```python
from build123d import *

# Parameters (mm, degrees)
REVOLVE1_ANGLE      = 180
SKETCH4_R           = 50
BOSS_EXTRUDE1_DEPTH = 7
SKETCH5_R           = 4
SKETCH5_R_2         = 1.5
BOSS_EXTRUDE2_DEPTH = 10
SKETCH6_R           = 27.5
CUT_EXTRUDE1_DEPTH  = 10
BOSS_EXTRUDE3_DEPTH = 7
SKETCH8_R           = 3
BOSS_EXTRUDE4_DEPTH = 15
BOSS_EXTRUDE5_DEPTH = 10


with BuildPart() as part:
    # Sketch1 → Revolve1 (revolve)
    with BuildSketch(Plane(origin=(0, 0, 0), x_dir=(1, 0, 0), z_dir=(0, 1, 0))):
        with BuildLine():
            Line((1.491717845, 54.979766986), (-1.491717845, -54.979766986))
            ThreePointArc((-1.491717845, -54.979766986), (54.979766986, -1.491717845), (1.491717845, 54.979766986))
        make_face()
    revolve(axis=Axis((1.491717845, 0, -54.979766986), (-0.027122143, 0, 0.999632127)), revolution_arc=REVOLVE1_ANGLE)

    # Sketch2 → Cut-Revolve1 (revolve, cut)
    with BuildSketch(Plane.XZ):
        with BuildLine():
            Line((49.980692072, 1.389395568), (-49.980692072, -1.389395568))
            ThreePointArc((-49.980692072, -1.389395568), (-1.389395568, 49.980692072), (49.980692072, 1.389395568))
        make_face()
    revolve(axis=Axis((49.980692072, 0, 1.389395568), (-0.999613841, 0, -0.027787911)), mode=Mode.SUBTRACT)

    # Sketch4 → Boss-Extrude1 (add)
    with BuildSketch(Plane.XZ):
        Circle(SKETCH4_R)
    extrude(amount=-BOSS_EXTRUDE1_DEPTH)

    # Sketch5 → Boss-Extrude2 (add)
    with BuildSketch(Plane.XZ):
        with Locations((0, 35)):
            Circle(SKETCH5_R)
        with Locations((0, 35)):
            Circle(SKETCH5_R_2, mode=Mode.SUBTRACT)
        with Locations((30.310889132, -17.5)):
            Circle(SKETCH5_R)
        with Locations((30.310889132, -17.5)):
            Circle(SKETCH5_R_2, mode=Mode.SUBTRACT)
        with Locations((-30.310889132, -17.5)):
            Circle(SKETCH5_R)
        with Locations((-30.310889132, -17.5)):
            Circle(SKETCH5_R_2, mode=Mode.SUBTRACT)
    extrude(amount=BOSS_EXTRUDE2_DEPTH)

    # Sketch6 → Cut-Extrude1 (cut)
    with BuildSketch(Plane.XZ):
        Circle(SKETCH6_R)
    extrude(amount=-CUT_EXTRUDE1_DEPTH, mode=Mode.SUBTRACT)

    # Sketch7 → Boss-Extrude3 (add)
    with BuildSketch(Plane.XZ):
        with BuildLine():
            Line((-29.59626463, 3), (-6.873863542, 3))
            ThreePointArc((-6.873863542, 3), (-5.303300859, 5.303300859), (-3, 6.873863542))
            Line((-3, 6.873863542), (-3, 29.076054117))
            Line((-3, 29.076054117), (3, 29.076054117))
            Line((3, 29.076054117), (3, 6.873863542))
            ThreePointArc((3, 6.873863542), (5.303300859, 5.303300859), (6.873863542, 3))
            Line((6.873863542, 3), (29.260564873, 3))
            Line((29.260564873, 3), (29.260564873, -3))
            Line((29.260564873, -3), (6.873863542, -3))
            ThreePointArc((6.873863542, -3), (5.303300859, -5.303300859), (3, -6.873863542))
            Line((3, -6.873863542), (3, -30.682999102))
            Line((3, -30.682999102), (-3, -30.682999102))
            Line((-3, -30.682999102), (-3, -6.873863542))
            ThreePointArc((-3, -6.873863542), (-5.303300859, -5.303300859), (-6.873863542, -3))
            Line((-6.873863542, -3), (-29.59626463, -3))
            Line((-29.59626463, -3), (-29.59626463, 3))
        make_face()
    extrude(amount=-BOSS_EXTRUDE3_DEPTH)

    # Sketch8 → Boss-Extrude4 (add)
    with BuildSketch(Plane.XZ):
        Circle(SKETCH8_R)
    extrude(amount=BOSS_EXTRUDE4_DEPTH)

    # Sketch9 → Boss-Extrude5 (add)
    with BuildSketch(Plane.XZ):
        Polygon((1, 1), (4.3, 1), (4.3, -1), (1, -1), (1, -4.3), (-1, -4.3), (-1, -1), (-4.3, -1), (-4.3, 1), (-1, 1), (-1, 4.3), (1, 4.3), align=None)
    extrude(amount=BOSS_EXTRUDE5_DEPTH)


solid = part.part
```
Input: part model. Units: mm. Frame: model coordinates. A direction names the side the tool comes from. Round coordinates to 2 decimals unless told otherwise and drop trailing zeros. Write each loop counter-clockwise with the first axis right and the second up, starting at its lowest first coordinate (ties: lowest second). Pieces come first, ordered by that corner, then holes. Notation, with made-up numbers: (-30.5, -24.5) - (14.5, -24.5) arc R23 ccw to (14.5, -1.5) - close; hole circle Ø11 at (61.25, -8). An arc over 180 degrees is marked (long way). Write item = value, one per line.
(1) Section query C-C on x = -15. Output: boundary loops of the cut face in (y, z), then the cut area to 3 significant figures.
Geometry check:
outline = (0, -52.92) arc R52.92 ccw to (0, 52.92) - (0, 23.05) - (7, 23.05) - (7, 47.18) arc R47.7 cw to (7, -47.18) - (7, -23.05) - (0, -23.05) - close; (0, -3) - (7, -3) - (7, 3) - (0, 3) - close
area = 1,210 mm^2
(2) Material intervals for probe 1 along Z at (x, y) = (0, -5); probe 2 along X at (y, z) = (4.5, -17); probe 3 along X at (y, z) = (-4, -17), sorted ascending.
Geometry check:
probe_1 = -4.3 to 4.3, 31 to 33.5, 36.5 to 39
probe_2 = -52.11 to -21.62, -3 to 3, 21.62 to 52.11
probe_3 = -34.28 to -31.73, -28.9 to -26.34, 26.34 to 28.9, 31.73 to 34.28
(3) Section query B-B on z = 35. Output: boundary loops of the cut face in (x, y).
Geometry check:
outline = (-42.43, 0) - (-4, 0) - (-4, -10) - (-1.5, -10) - (-1.5, 0) - (1.5, 0) - (1.5, -10) - (4, -10) - (4, 0) - (42.43, 0) arc R42.43 ccw to start; hole (-35.01, 7) - (35.01, 7) arc R35.71 ccw to start
(4) Access query for faces 1 (the flat face through (1, 7, 1)), 2 (the flat face through (2, -10, 35)), 3 (the cylindrical face through (-0.325, -4.93, 33.536)), 4 (the flat face through (32, -10, -17)). Directions: +Z, -Z, +X, -X, +Y, -Y. A direction counts if a zero-diameter tool reaches every point of the face in a straight line with its end or side. Return the directions, or none.
Geometry check:
face_1 = none
face_2 = +Z, +X, -X, -Y
face_3 = -Y
face_4 = +Z, -Z, +X, -X, -Y
(5) Section query A-A on z = -17.5. Output: boundary loops of the cut face in (x, y).
Geometry check:
outline = (-52.14, 0) - (-34.31, 0) - (-34.31, -10) - (-31.81, -10) - (-31.81, 0) - (-28.81, 0) - (-28.81, -10) - (-26.31, -10) - (-26.31, 0) - (-21.21, 0) - (-21.21, 7) - (-46.31, 7) arc R46.84 cw to (46.31, 7) - (21.21, 7) - (21.21, 0) - (26.31, 0) - (26.31, -10) - (28.81, -10) - (28.81, 0) - (31.81, 0) - (31.81, -10) - (34.31, -10) - (34.31, 0) - (52.14, 0) arc R52.14 ccw to start; (-3, 0) - (3, 0) - (3, 7) - (-3, 7) - close
(6) Section query D-D on y = 46.5. Output: boundary loops of the cut face in (x, z), then the cut area to 3 significant figures.
Geometry check:
outline = circle Ø58.75 at (0, 0); hole circle Ø36.76 at (0, 0)
area = 1,650 mm^2
(7) Pull-direction query (X, two-part tool) for faces 5 (the cylindrical face through (19.63, 3.45, 19.26)), 6 (the cylindrical face through (19.26, 3.45, -19.63)), 7 (the flat face through (-30.4, -10, -19.2)); classes: +X half, -X half, draft (parallel to the pull), parting line (faces both ways), or undercut.
Geometry check:
face_5 = undercut
face_6 = undercut
face_7 = draft
(8) Contact query for flat-ended pins moving along their axis: pin 1 Ø0.7 at (x, z) = (-0.5, -3.5) entering from -Y; pin 2 Ø1.2 at (x, y) = (-3.5, -5.5) entering from -Z; pin 3 Ø6 at (y, z) = (3, -35.5) entering from +X. Output: stop coordinate, or through.
Geometry check:
pin_1 = -10
pin_2 = -1
pin_3 = 44.28
